```python
from build123d import *

# Parameters (mm, degrees)
SKIZZE1_W                       = 16.8
SKIZZE1_H                       = 3
SKIZZE2_R                       = 1
SCHNITT_LINEAR_AUSTRAGEN1_DEPTH = 4
KREISMUSTER1_COUNT              = 3
M4_GEWINDEBOHRUNG1_D            = 3.3


with BuildPart() as part:
    # Skizze1 → Rotation1 (revolve)
    with BuildSketch(Plane(origin=(0, 0, 0), x_dir=(0, 0, -1), z_dir=(1, 0, 0))):
        with Locations((-9.4, 1.5)):
            Rectangle(SKIZZE1_W, SKIZZE1_H)
    revolve(axis=Axis((0, 0, 0), (0, 1, 0)))

    # Skizze2 → Schnitt-Linear austragen1 (cut, through all)
    with BuildSketch(Plane(origin=(0, 3, 0), x_dir=(1, 0, 0), z_dir=(0, 1, 0))):
        with Locations((-12, 0)):
            Circle(SKIZZE2_R)
    schnitt_linear_austragen1 = extrude(amount=-SCHNITT_LINEAR_AUSTRAGEN1_DEPTH, mode=Mode.SUBTRACT)

    # Kreismuster1: Schnitt-Linear austragen1 ×3 about axis
    kreismuster1_axis = Axis((0, 0, 0), (0, 1, 0))
    for i in range(1, KREISMUSTER1_COUNT):
        add(schnitt_linear_austragen1.rotate(kreismuster1_axis, i * 360 / KREISMUSTER1_COUNT), mode=Mode.SUBTRACT)

    # M4 Gewindebohrung1 (through all)
    with Locations(Plane(origin=(0, 3, 0), x_dir=(1, 0, 0), z_dir=(0, 1, 0))):
        with Locations((0, 0), (6, 10.392304845), (-12, 0), (6, -10.392304845)):
            Hole(M4_GEWINDEBOHRUNG1_D / 2)


solid = part.part
```
Input: part model. Units: mm. Frame: model coordinates. Give positions to 0.01 mm unless a question says otherwise; leave off trailing zeros. Order: outer loops, then holes, each group sorted by start corner. A loop starts at its lowest first (then second) coordinate and runs counter-clockwise, first axis right, second up. Notation, with made-up numbers: (-14, 84) - (4, 84) arc R33 cw to (4, 121) - close; hole circle Ø3 at (-1, -9.5). An arc over 180 degrees is marked (long way). Use a Markdown table: item, result.
(1) Pin query (flat end, axial travel): pin 1 (1 mm diameter, centred on x = -9, y = 1.5, fed in from -Z). Return the tip coordinate at first contact, or that it passes through.
Computed values:
| item | result |
|---|---|
| pin 1 | stops at z = -15.64 |
(2) Draft query along Z for faces 1 (the flat face through (0, 3, 4)), 2 (the cylindrical face through (-17.377, 1.521, -3.859)), 3 (the cylindrical face through (7.309, 1.479, 11.396)). Return one class per face: released by +Z, released by -Z, zero draft, split by the parting line, or undercut.
Computed values:
| item | result |
|---|---|
| face 1 | zero draft |
| face 2 | split by the parting line |
| face 3 | undercut |
(3) Section query D-D (y = 0.5). Output: boundary loops of the cut face in (x, z), then the cut area to 3 significant figures.
Computed values:
| item | result |
|---|---|
| outline | circle Ø35.6 at (0, 0); hole circle Ø3.3 at (-12, 0); hole circle Ø3.3 at (0, 0); hole circle Ø3.3 at (6, -10.39); hole circle Ø3.3 at (6, 10.39) |
| area | 961 mm2 |
(4) Section query A-A (z = 0). Output: boundary loops of the cut face in (x, y), then the cut area to 3 significant figures.
Computed values:
| item | result |
|---|---|
| outline | (-17.8, 0) - (-13.65, 0) - (-13.65, 3) - (-17.8, 3) - close; (-10.35, 0) - (-1.65, 0) - (-1.65, 3) - (-10.35, 3) - close; (1.65, 0) - (17.8, 0) - (17.8, 3) - (1.65, 3) - close |
| area | 87.0 mm2 |
(5) Section query B-B (x = 0). Output: boundary loops of the cut face in (y, z).
Computed values:
| item | result |
|---|---|
| outline | (0, -17.8) - (3, -17.8) - (3, -1.65) - (0, -1.65) - close; (0, 1.65) - (3, 1.65) - (3, 17.8) - (0, 17.8) - close |
(6) Section query C-C (x = 6). Output: boundary loops of the cut face in (y, z), then the cut area to 3 significant figures.
Computed values:
| item | result |
|---|---|
| outline | (0, -16.76) - (3, -16.76) - (3, -12.04) - (0, -12.04) - close; (0, -8.74) - (3, -8.74) - (3, 8.74) - (0, 8.74) - close; (0, 12.04) - (3, 12.04) - (3, 16.76) - (0, 16.76) - close |
| area | 80.7 mm2 |
(7) Line query: line 1 (Z direction, x = 6, y = 2.35); line 2 (X direction, y = 1.2, z = -1.5); line 3 (X direction, y = 0.7, z = -1). Output: solid intervals per line, ascending. Write a range as from..to.
Computed values:
| item | result |
|---|---|
| line 1 | z = -16.76..-12.04, -8.74..8.74, 12.04..16.76 |
| line 2 | x = -17.74..-12.69, -11.31..-0.69, 0.69..17.74 |
| line 3 | x = -17.77..-13.31, -10.69..-1.31, 1.31..17.77 |
